```python
from build123d import *

# Parameters (mm, degrees)
SKETCH1_W                = 76.2
SKETCH1_H                = 50.8
BOSS_EXTRUDE1_DEPTH      = 31.75
BOSS_EXTRUDE2_DEPTH      = 31.75
BOSS_EXTRUDE2_DEPTH_BACK = 85.09
SKETCH4_W                = 5.08
SKETCH4_H                = 2.54
SKETCH4_W_2              = 7.62
SKETCH4_H_2              = 7.62
FILLET1_R                = 10.16
SKETCH5_W                = 7.62
SKETCH5_H                = 7.62
BOSS_EXTRUDE3_DEPTH      = 12.7
SKETCH6_W                = 7.62
SKETCH6_H                = 2.54
CUT_EXTRUDE1_DEPTH       = 7.62
SKETCH7_W                = 7.62
SKETCH7_H                = 2.54
CUT_EXTRUDE2_DEPTH       = 7.62
SKETCH9_W                = 7.62
SKETCH9_H                = 5.08
BOSS_EXTRUDE4_DEPTH      = 7.62
SKETCH10_W               = 7.62
SKETCH10_H               = 5.08
BOSS_EXTRUDE5_DEPTH      = 7.62
FILLET2_R                = 3.81
CUT_EXTRUDE3_REACH       = 116.166
SKETCH11_R               = 2.54
CUT_EXTRUDE4_REACH       = 116.166
SKETCH12_R               = 2.54
CUT_EXTRUDE5_REACH       = 145.06
SKETCH13_W               = 3.81
SKETCH13_H               = 0.635
SKETCH14_W               = 3.81
SKETCH14_H               = 0.635
CUT_EXTRUDE6_DEPTH       = 34.29


# Some blends are built 0.0001 mm under size
with BuildPart() as part:
    # Sketch1 → Boss-Extrude1 (new body)
    with BuildSketch(Plane.XY):
        with Locations((-38.1, 25.4)):
            Rectangle(SKETCH1_W, SKETCH1_H)
    extrude(amount=BOSS_EXTRUDE1_DEPTH)

    # Sketch4 → Boss-Extrude2 (add, two sides: drawn at the far end of the back side and taken through both)
    with BuildSketch(Plane(origin=(0, 50.8, 0), x_dir=(1, 0, 0), z_dir=(0, 1, 0)).offset(-BOSS_EXTRUDE2_DEPTH_BACK)):
        with Locations((-58.42, -8.89)):
            Rectangle(SKETCH4_W, SKETCH4_H)
        with Locations((-46.99, -3.81)):
            Rectangle(SKETCH4_W_2, SKETCH4_H_2)
    extrude(amount=BOSS_EXTRUDE2_DEPTH + BOSS_EXTRUDE2_DEPTH_BACK)

    # Fillet1
    # the kernel refuses this fillet: 10.16 mm, written as the material it adds along each edge
    with BuildSketch(Plane(origin=(-50.8, 50.8, 7.62), x_dir=(-1, 0, 0), z_dir=(0, 0, -1)), Plane(origin=(-50.8, 0, 0), x_dir=(-1, 0, 0), z_dir=(0, 0, 1))) as fillet1_piece_1:
        with BuildLine():
            CenterArc((FILLET1_R, FILLET1_R), FILLET1_R, 180, 90)
            Line((0, FILLET1_R), (0, 0))
            Line((0, 0), (FILLET1_R, 0))
        make_face()
    extrude(amount=7.62)

    # Sketch5 → Boss-Extrude3 (add)
    with BuildSketch(Plane.XY.offset(7.62)):
        with Locations((-46.99, 71.12)):
            Rectangle(SKETCH5_W, SKETCH5_H)
        with Locations((-46.99, -22.86)):
            Rectangle(SKETCH5_W, SKETCH5_H)
    extrude(amount=BOSS_EXTRUDE3_DEPTH)

    # Sketch6 → Cut-Extrude1 (cut)
    with BuildSketch(Plane.XZ.offset(34.29)):
        with Locations((-46.99, 6.35)):
            Rectangle(SKETCH6_W, SKETCH6_H)
    extrude(amount=-CUT_EXTRUDE1_DEPTH, mode=Mode.SUBTRACT)

    # Sketch7 → Cut-Extrude2 (cut)
    with BuildSketch(Plane(origin=(0, 82.55, 0), x_dir=(1, 0, 0), z_dir=(0, 1, 0))):
        with Locations((-46.99, -6.35)):
            Rectangle(SKETCH7_W, SKETCH7_H)
    extrude(amount=-CUT_EXTRUDE2_DEPTH, mode=Mode.SUBTRACT)

    # Sketch9 → Boss-Extrude4 (add)
    with BuildSketch(Plane(origin=(0, -26.67, 0), x_dir=(-1, 0, 0), z_dir=(0, -1, 0))):
        with Locations((46.99, -17.78)):
            Rectangle(SKETCH9_W, SKETCH9_H)
    extrude(amount=BOSS_EXTRUDE4_DEPTH)

    # Sketch10 → Boss-Extrude5 (add)
    with BuildSketch(Plane(origin=(0, 74.93, 0), x_dir=(1, 0, 0), z_dir=(0, 1, 0))):
        with Locations((-46.99, -17.78)):
            Rectangle(SKETCH10_W, SKETCH10_H)
    extrude(amount=BOSS_EXTRUDE5_DEPTH)

    # Fillet2
    fillet2_edges = [part.edges().sort_by_distance(p)[0] for p in [
        (-43.18, 82.55, 2.54),
        (-50.8, 82.55, 2.54),
        (-43.18, 82.55, 17.78),
        (-50.8, 82.55, 17.78),
        (-50.8, -34.29, 2.54),
        (-43.18, -34.29, 2.54),
        (-50.8, -34.29, 17.78),
        (-43.18, -34.29, 17.78),
    ]]
    fillet(fillet2_edges, radius=FILLET2_R - 0.0001)  # a hair under: the kernel refuses the full size

    # Cut-Extrude3: up to this face of the body (flat: up to its plane)
    cut_extrude3_end = Plane(part.part.faces().sort_by_distance((-39.240735796, 25.146964219, 0))[0])
    # Sketch11 → Cut-Extrude3 (cut, up to the picked face)
    with BuildSketch(Plane.XY.offset(20.32), mode=Mode.PRIVATE) as cut_extrude3_sk1:
        with Locations((-46.99, 78.74)):
            Circle(SKETCH11_R)
    cut_extrude3_tool1 = split(extrude(cut_extrude3_sk1.sketch, amount=-CUT_EXTRUDE3_REACH, mode=Mode.PRIVATE), bisect_by=cut_extrude3_end, keep=Keep.BOTH, mode=Mode.PRIVATE)
    add(cut_extrude3_tool1.solids().sort_by(Axis((-46.99, 78.74, 20.32), (0, 0, -1)))[0], mode=Mode.SUBTRACT)

    # Cut-Extrude4: up to this face of the body (flat: up to its plane)
    cut_extrude4_end = Plane(part.part.faces().sort_by_distance((-39.204923448, 24.89929007, 0))[0])
    # Sketch12 → Cut-Extrude4 (cut, up to the picked face)
    with BuildSketch(Plane.XY.offset(20.32), mode=Mode.PRIVATE) as cut_extrude4_sk1:
        with Locations((-46.99, -30.48)):
            Circle(SKETCH12_R)
    cut_extrude4_tool1 = split(extrude(cut_extrude4_sk1.sketch, amount=-CUT_EXTRUDE4_REACH, mode=Mode.PRIVATE), bisect_by=cut_extrude4_end, keep=Keep.BOTH, mode=Mode.PRIVATE)
    add(cut_extrude4_tool1.solids().sort_by(Axis((-46.99, -30.48, 20.32), (0, 0, -1)))[0], mode=Mode.SUBTRACT)

    # Cut-Extrude5: up to this face of the body (flat: up to its plane)
    cut_extrude5_end = Plane(part.part.faces().sort_by_distance((-37.151107955, 50.8, 16.634474432))[0])
    # Sketch13 → Cut-Extrude5 (cut, up to the picked face)
    with BuildSketch(Plane(origin=(0, 82.55, 0), x_dir=(1, 0, 0), z_dir=(0, 1, 0)), mode=Mode.PRIVATE) as cut_extrude5_sk1:
        with Locations((-58.42, -9.8425)):
            Rectangle(SKETCH13_W, SKETCH13_H)
    cut_extrude5_tool1 = split(extrude(cut_extrude5_sk1.sketch, amount=-CUT_EXTRUDE5_REACH, mode=Mode.PRIVATE), bisect_by=cut_extrude5_end, keep=Keep.BOTH, mode=Mode.PRIVATE)
    # Sketch13 → Cut-Extrude5 (cut, up to the picked face)
    with BuildSketch(Plane(origin=(0, 82.55, 0), x_dir=(1, 0, 0), z_dir=(0, 1, 0)), mode=Mode.PRIVATE) as cut_extrude5_sk2:
        with Locations((-58.42, -7.9375)):
            Rectangle(SKETCH13_W, SKETCH13_H)
    cut_extrude5_tool2 = split(extrude(cut_extrude5_sk2.sketch, amount=-CUT_EXTRUDE5_REACH, mode=Mode.PRIVATE), bisect_by=cut_extrude5_end, keep=Keep.BOTH, mode=Mode.PRIVATE)
    add(cut_extrude5_tool1.solids().sort_by(Axis((-58.42, 82.55, 9.8425), (0, -1, 0)))[0], mode=Mode.SUBTRACT)
    add(cut_extrude5_tool2.solids().sort_by(Axis((-58.42, 82.55, 7.9375), (0, -1, 0)))[0], mode=Mode.SUBTRACT)

    # Sketch14 → Cut-Extrude6 (cut)
    with BuildSketch(Plane(origin=(0, -34.29, 0), x_dir=(-1, 0, 0), z_dir=(0, -1, 0))):
        with Locations((58.42, -9.8425)):
            Rectangle(SKETCH14_W, SKETCH14_H)
        with Locations((58.42, -7.9375)):
            Rectangle(SKETCH14_W, SKETCH14_H)
    extrude(amount=-CUT_EXTRUDE6_DEPTH, mode=Mode.SUBTRACT)


solid = part.part
```
Work out the finished part from the listing and answer in its coordinate system (mm). A direction names the side the tool comes from. Coordinates: 2 decimals unless noted, no trailing zeros. Loops run counter-clockwise (first coordinate to the right, second up) from the corner with the lowest first, then second, coordinate; pieces in that order, holes last.
1) Flat-ended cylindrical pins translate along their axes: pin 1 (1.3 mm diameter, centred on y = 69.5, z = 9, fed in from +X); pin 2 (0.5 mm diameter, centred on x = -56, y = 61, fed in from -Z); pin 3 (6 mm diameter, centred on x = -59, y = 63, fed in from +Z). Find the tip coordinate at first contact, or state that the pin passes through.
Results:
pin 1: stops at x = -43.18
pin 2: stops at z = 7.62
pin 3: stops at z = 10.16
2) Consider probe 1 along Y at (x, z) = (-46.99, 2.3); probe 2 along Y at (x, z) = (-46.99, 17.5); probe 3 along Y at (x, z) = (-46, 1). Determine where each line is inside the solid, lowest interval first.
Results:
probe 1: y = -34.29 to -33.02, -27.94 to 76.2, 81.28 to 82.55
probe 2: y = -34.29 to -33.02, -27.94 to -19.05, 0 to 50.8, 67.31 to 76.2, 81.28 to 82.55
probe 3: y = -34.16 to -32.82, -28.14 to 76.4, 81.08 to 82.42
3) For a pull along Z with two mould halves and no side action, classify faces 1 (the flat face through (-46, 76, 5.08)), 2 (the cylindrical face through (-44.266, 81.404, 2.504)), 3 (the flat face through (-39, 25, 0)) as +Z half, -Z half, draft (parallel to the pull), parting line (faces both ways), or undercut.
Results:
face 1: undercut
face 2: draft
face 3: -Z half
4) Section A-A (y = -24) is taken. Give the vertices of the cut face in (x, z) (3 decimals).
Results:
outline: (-60.96, 7.62) - (-60.325, 7.62) - (-60.325, 8.255) - (-56.515, 8.255) - (-56.515, 7.62) - (-55.88, 7.62) - (-55.88, 10.16) - (-56.515, 10.16) - (-56.515, 9.525) - (-60.325, 9.525) - (-60.325, 10.16) - (-60.96, 10.16) - close; (-50.8, 0) - (-43.18, 0) - (-43.18, 20.32) - (-50.8, 20.32) - close
5) For faces 4 (the flat face through (-43.18, 68, 8)), 5 (the flat face through (-60.96, -17, 9)), 6 (the flat face through (-47, 67.31, 14)), determine the directions among +Z, -Z, +X, -X, +Y, -Y from which every point of the face is accessible in a straight line to the end or side of a thin tool.
Results:
face 4: +Z, -Z, +X, +Y
face 5: +Z, -Z, -X, -Y
face 6: +Z, +X
6) Section B-B (x = -65) is taken. Give the vertices of the cut face in (y, z).
Results:
outline: (0, 0) - (50.8, 0) - (50.8, 31.75) - (0, 31.75) - close
